from build123d import *

# Parameters (mm, degrees)
SKETCH1_R           = 3.5
SKETCH1_R_2         = 2.25
BOSS_EXTRUDE1_DEPTH = 2
SKETCH2_R           = 1.25
SKETCH2_R_2         = 0.5
BOSS_EXTRUDE3_DEPTH = 2


with BuildPart() as part:
    # Sketch1 → Boss-Extrude1 (new body)
    with BuildSketch(Plane(origin=(0, 0, 0), x_dir=(1, 0, 0), z_dir=(0, 1, 0))):
        Circle(SKETCH1_R)
        Circle(SKETCH1_R_2, mode=Mode.SUBTRACT)
    extrude(amount=BOSS_EXTRUDE1_DEPTH)

    # Sketch2 → Boss-Extrude3 (add)
    with BuildSketch(Plane(origin=(0, 2, 0), x_dir=(1, 0, 0), z_dir=(0, 1, 0))):
        with BuildLine():
            Line((-7.000925654, 1.878025645), (-6.999074346, -1.878025645))
            Line((-6.999074346, -1.878025645), (0, -3.5))
            ThreePointArc((0, -3.5), (3.5, 0), (0, 3.5))
            Line((0, 3.5), (-7.000925654, 1.878025645))
        make_face()
        Circle(SKETCH2_R, mode=Mode.SUBTRACT)
        with Locations((-5, 0)):
            Circle(SKETCH2_R_2, mode=Mode.SUBTRACT)
    extrude(amount=BOSS_EXTRUDE3_DEPTH)


solid = part.part
Input: part model. Units: mm. Frame: model coordinates. A direction names the side the tool comes from. Coordinates: 2 decimals unless noted, no trailing zeros. Order: outer loops, then holes, each group sorted by start corner. A loop starts at its lowest first (then second) coordinate and runs counter-clockwise, first axis right, second up. Notation, with made-up numbers: M -33,-30.75 L -16,-30.75 A22 ccw -16,3.25 Z; hole C 62.25,10.25 d11. An arc over 180 degrees is marked long. Answer in a Markdown table with one row per item.
(1) Material intervals for line 1 (X direction, y = 3.5, z = 0); line 2 (X direction, y = 1.25, z = 0), sorted ascending. Write a range as [from, to].
Numbers:
| item | result |
|---|---|
| line 1 | x = [-7, -5.5], [-4.5, -1.25], [1.25, 3.5] |
| line 2 | x = [-3.5, -2.25], [2.25, 3.5] |
(2) Section query D-D, the plane y = 2.7. Output: boundary loops of the cut face in (x, z).
Numbers:
| item | result |
|---|---|
| outline | M -7,-1.88 L 0,-3.5 A3.5 ccw 0,3.5 L -7,1.88 Z; hole C -5,0 d1; hole C 0,0 d2.5 |
(3) Access query for faces 1 (the flat face through (-3.45, 2.99, -2.7)), 2 (the cylindrical face through (-0.27, 2.99, 1.22)), 3 (the flat face through (1, 2, 1)). Directions: +Z, -Z, +X, -X, +Y, -Y. A direction counts if a zero-diameter tool reaches every point of the face in a straight line with its end or side. Return the directions, or none.
Numbers:
| item | result |
|---|---|
| face 1 | -Z, -X, +Y |
| face 2 | +Y, -Y |
| face 3 | -Y |
(4) Section query C-C, the plane z = 0.75. Output: boundary loops of the cut face in (x, y), plus the area to 3 significant figures.
Numbers:
| item | result |
|---|---|
| outline | M -7,2 L -3.42,2 L -3.42,0 L -2.12,0 L -2.12,2 L -1,2 L -1,4 L -7,4 Z; M 1,2 L 2.12,2 L 2.12,0 L 3.42,0 L 3.42,4 L 1,4 Z |
| area | 22.0 mm^2 |
(5) Draft query along X for faces 4 (the flat face through (0.7, 0, 2.3)), 5 (the cylindrical face through (3.086, 2.416, 1.651)), 6 (the cylindrical face through (-5.4, 3, 0.3)), 7 (the flat face through (-3.549, 2.986, 2.678)). Return one class per face: pulls with the +X half, pulls with the -X half, needs draft (parallel to the pull), parting line crosses it, or undercut.
Numbers:
| item | result |
|---|---|
| face 4 | needs draft |
| face 5 | parting line crosses it |
| face 6 | undercut |
| face 7 | pulls with the -X half |
(6) Section query A-A, the plane z = 0. Output: boundary loops of the cut face in (x, y), plus the area to 3 significant figures.
Numbers:
| item | result |
|---|---|
| outline | M -7,2 L -5.5,2 L -5.5,4 L -7,4 Z; M -4.5,2 L -3.5,2 L -3.5,0 L -2.25,0 L -2.25,2 L -1.25,2 L -1.25,4 L -4.5,4 Z; M 1.25,2 L 2.25,2 L 2.25,0 L 3.5,0 L 3.5,4 L 1.25,4 Z |
| area | 19.0 mm^2 |
(7) Section query B-B, the plane x = -5. Output: boundary loops of the cut face in (y, z), plus the area to 3 significant figures.
Numbers:
| item | result |
|---|---|
| outline | M 2,-2.34 L 4,-2.34 L 4,-0.5 L 2,-0.5 Z; M 2,0.5 L 4,0.5 L 4,2.34 L 2,2.34 Z |
| area | 7.37 mm^2 |
(8) Contact query for flat-ended pins moving along their axis: pin 1 Ø2 at (y, z) = (1, 2.5) entering from +X; pin 2 Ø2 at (x, z) = (-6, 2.5) entering from -Y; pin 3 Ø1 at (y, z) = (1.5, 1) entering from +X. Output: stop coordinate, or through.
Numbers:
| item | result |
|---|---|
| pin 1 | stops at x = 3.16 |
| pin 2 | stops at y = 2 |
| pin 3 | stops at x = 3.46 |
